Can you work these out from the model? Positions are in its coordinate system, mm. A direction names the side the tool comes from. Give positions to 0.01 mm unless a question says otherwise; leave off trailing zeros. Loops run counter-clockwise (first coordinate to the right, second up) from the corner with the lowest first, then second, coordinate; pieces in that order, holes last. Notation, with made-up numbers: (44, 68) - (82, 68) arc R30 ccw to (82, 93) - close; hole circle Ø1 at (67, 71). An arc over 180 degrees is marked (long way). Answer in a Markdown table with one row per item.
Autodesk Inventor part; units mm, degrees
ref_plane "Work Plane2" through (0, 0, 5) normal (0, 0, 1) x (1, 0, 0)
ref_plane "Work Plane8" through (0, 0, 0) normal (0.9238795, 0.3826834, 0) x (0, 0, 1)
ref_plane "Work Plane9" through (0, 0, 0) normal (1, 0, 0) x (0, 1, 0)
sketch "Sketch1" plane through (0, 0, 0) normal (0, 0, 1) x (1, 0, 0)
  circle A0 centre (0, 0) radius 6.25
  dimension "d0" = 12.5
extrude "Extrusion1" add sketch "Sketch1" along normal blind 10
ref_plane "Work Plane2" through (0, 0, 5) normal (0, 0, 1) x (1, 0, 0)
sketch "Sketch2" plane through (0, 0, 0) normal (0, 0, -1) x (-1, 0, 0)
  circle A0 centre (0, 0) radius 6.25
  circle A1 centre (0, 0) radius 5
  dimension "d3" = 10
surface extrude "Pitch Diameter" sketch "Sketch2" against normal through all shown no curves A1
ref_plane "Work Plane8" through (0, 0, 0) normal (0.9238795, 0.3826834, 0) x (0, 0, 1)
ref_plane "Work Plane9" through (0, 0, 0) normal (1, 0, 0) x (0, 1, 0)
spur gear teeth "Spur Gear" teeth 8 pitch diameter 10 tip diameter 12.5 root diameter 6.875 face width 10 start plane through (0, 0, 0) normal (0, 0, -1) x (-1, 0, 0)
sketch "Sketch3" plane through (0, 0, 10) normal (0, 0, 1) x (1, 0, 0)
  arc A0 (-3.965, 4.8313) -> (-4.8313, 3.965) centre (0, 0) ccw
  circle A1 centre (0, 0) radius 1.5
  dimension "d49" = 3
extrude "Extrusion2" cut sketch "Sketch3" against normal blind 30
equation "\"d0\" = da_da"
equation "\"d1\" = da_b"
equation "\"d3\" = da_dw"
equation "\"d16\" = da_aw"
equation "\"d43\" = da_aw"
equation "\"d46\" = da_aw"
properties part number "Spur Gear1" material "Steel"
Q1. If we mould it in two halves opening along Y, with no side actions, what happens to faces 5 (the face through (-6.25, -0.01, 4.93)), 6 (the face through (-4.1, -2.7, 4.9)), 7 (the face through (-4.41, -4.43, 4.93))? For each: released by +Y, released by -Y, zero draft, split by the parting line, or undercut.
Checked values:
| item | result |
|---|---|
| face 5 | split by the parting line |
| face 6 | undercut |
| face 7 | released by -Y |
Q2. Imagine slicing it at A-A, the plane y = 0. Write out the boundary of the cut face in (x, z), and give its area (3 significant figures).
Checked values:
| item | result |
|---|---|
| outline | (-6.25, 0) - (-1.5, 0) - (-1.5, 10) - (-6.25, 10) - close; (1.5, 0) - (6.25, 0) - (6.25, 10) - (1.5, 10) - close |
| area | 95.0 mm² |
Q3. Imagine slicing it at D-D, the plane y = -2.5. Write out the boundary of the cut face in (x, z).
Checked values:
| item | result |
|---|---|
| outline | (-3.94, 0) - (3.94, 0) - (3.94, 10) - (-3.94, 10) - close |
Q4. If I drill on line 1 (X direction, y = 4.5, z = 3.25); line 2 (Y direction, x = 0, z = 3.75); line 3 (X direction, y = 4.75, z = 2.25), over which ranges is the centre line in solid material (lowest first)? Write a range as [from, to].
Checked values:
| item | result |
|---|---|
| line 1 | x = [-4.34, -3.3], [-1.02, 1.02], [3.3, 4.34] |
| line 2 | y = [-6.25, -1.5], [1.5, 6.25] |
| line 3 | x = [-4.06, -3.78], [-1, 1], [3.78, 4.06] |
Q5. On a 3-axis mill with a long thin cutter (end or side, diameter ignored), from which of +Z, -Z, +X, -X, +Y, -Y can I reach the whole of each face in a straight line? I mean faces 1 (the face through (-4.8, 0.99, 4.93)), 2 (the face through (-2.7, -4.1, 4.9)), 3 (the face through (-4.1, 2.7, 4.9)), 4 (the face through (4.1, -2.7, 4.9)). Say none if no direction works.
Checked values:
| item | result |
|---|---|
| face 1 | +Z, -Z |
| face 2 | +Z, -Z, -Y |
| face 3 | +Z, -Z, -X |
| face 4 | +Z, -Z, +X |
